Check sheet for the modelled part. Datum: model origin and axes. Units: mm. Round coordinates to 2 decimals unless told otherwise and drop trailing zeros. Order: outer loops, then holes, each group sorted by start corner. A loop starts at its lowest first (then second) coordinate and runs counter-clockwise, first axis right, second up.
(1) Sectioned sample at A-A, the plane y = 4. Enter the section's corners in (x, z).
(2) Depth check by flat-ended pin: pin 1 (8 mm diameter, centred on y = 4.5, z = 760.5, fed in from +X); pin 2 (8 mm diameter, centred on x = 18, z = 262.5, fed in from -Y); pin 3 (1 mm diameter, centred on x = 16, z = 714, fed in from +Y). Enter the tip coordinate at first touch or a pass-through.
(3) Thickness scan on probe 1 along Z at (x, y) = (38, 0.5); probe 2 along Z at (x, y) = (4, -6); probe 3 along Z at (x, y) = (30, -5.5). Record the ranges inside material, lowest first.
```python
from build123d import *

# Parameters (mm, degrees)
F0_W         = 20
F0_H         = 1249.13
F0_W_2       = 50
F0_H_2       = 16
F0_H_3       = 2
F1_DEPTH     = 10
F0_H_4       = 19
F2_DEPTH     = 11.5
F3_DEPTH     = 9.5
F4_DEPTH     = 8
F5_R         = 7.99999
F6_R         = 9.49999
F7_T1_DEPTH  = 107.4995000022
F7_T6_DEPTH  = 107.4995000022
F7_T12_DEPTH = 107.4995000022
F7_T18_DEPTH = 107.4995000022
F7_T25_DEPTH = 107.4995000022
F7_T31_DEPTH = 107.4995000022
F7_T37_DEPTH = 107.4995000022
F7_T43_DEPTH = 107.4995000022
F7_T49_DEPTH = 107.4995000022
F7_T56_DEPTH = 107.4995000022
F7_T62_DEPTH = 107.4995000022
F8_R         = 9.99999


# Not quite as in the source:
# - a fillet or chamfer that OpenCascade refuses, or shapes differently, is made with other operations: its cross-section is extruded or revolved along the edge and cut away or added
# - a fillet or chamfer is up to 0.001 mm smaller than in the source, because OpenCascade refuses the exact size


with BuildPart() as f1:
    # F0 (on Front) → F1 (new body, symmetric)
    with BuildSketch(Plane.XZ):
        with Locations((25, 647.565)):
            Rectangle(F0_W, F0_H)
        Polygon((0, 1272.13), (15, 1272.13), (35, 1272.13), (50, 1272.13), (50, 1274.13), (0, 1274.13), align=None)
        with Locations((25, 1282.13)):
            Rectangle(F0_W_2, F0_H_2)
        with Locations((25, 1291.13)):
            Rectangle(F0_W_2, F0_H_3)
    extrude(amount=F1_DEPTH, both=True)

    # F0 (on Front) → F2 (join, symmetric)
    with BuildSketch(Plane.XZ):
        Polygon((0, 23), (0, 21), (50, 21), (50, 23), (35, 23), (15, 23), align=None)
        with Locations((25, 11.5)):
            Rectangle(F0_W_2, F0_H_4)
        with Locations((25, 1)):
            Rectangle(F0_W_2, F0_H_3)
    extrude(amount=F2_DEPTH, both=True)

    # F0 (on Front) → F3 (cut, symmetric)
    with BuildSketch(Plane.XZ):
        with Locations((25, 11.5)):
            Rectangle(F0_W_2, F0_H_4)
    extrude(amount=F3_DEPTH, both=True, mode=Mode.SUBTRACT)

    # F0 (on Front) → F4 (cut, symmetric)
    with BuildSketch(Plane.XZ):
        with Locations((25, 1282.13)):
            Rectangle(F0_W_2, F0_H_2)
    extrude(amount=F4_DEPTH, both=True, mode=Mode.SUBTRACT)

    # F5 (radius 8 in the source; OpenCascade refuses exactly that, so slightly less here)
    f5_edges = [f1.edges().sort_by_distance(p)[0] for p in [
        (25, -8, 1290.13),
        (25, -8, 1274.13),
        (25, 8, 1274.13),
        (25, 8, 1290.13),
    ]]
    fillet(f5_edges, radius=F5_R)

    # F6 (radius 9.5 in the source; OpenCascade refuses exactly that, so slightly less here)
    f6_edges = [f1.edges().sort_by_distance(p)[0] for p in [
        (25, 9.5, 2),
        (25, -9.5, 2),
        (25, -9.5, 21),
        (25, 9.5, 21),
    ]]
    fillet(f6_edges, radius=F6_R)

    # F7: fillet of radius 11.5 on 4 edges, made by hand

    # F7_s2 → F7_t1 (cut)
    with BuildSketch(Plane.YZ.offset(-28.7497500011)):
        with BuildLine():
            ThreePointArc((-0.0001, -0.0001), (-8.1318279836, 3.3681720164), (-11.5001, 11.4999))
            Line((-11.5001, 11.4999), (-11.7301, 11.4999))
            ThreePointArc((-11.7301, 11.4999), (-11.73, 5.74995), (-11.73, 0))
            Line((-11.73, 0), (-11.5, -0.23))
            ThreePointArc((-11.5, -0.23), (-5.75005, -0.23), (-0.0001, -0.2301))
            Line((-0.0001, -0.2301), (-0.0001, -0.0001))
        make_face()
        with BuildLine():
            ThreePointArc((0.0001, -0.0001), (8.1318279836, 3.3681720164), (11.5001, 11.4999))
            Line((11.5001, 11.4999), (11.7301, 11.4999))
            ThreePointArc((11.7301, 11.4999), (11.73, 5.74995), (11.73, 0))
            Line((11.73, 0), (11.5, -0.23))
            ThreePointArc((11.5, -0.23), (5.75005, -0.23), (0.0001, -0.2301))
            Line((0.0001, -0.2301), (0.0001, -0.0001))
        make_face()
    extrude(amount=F7_T1_DEPTH, mode=Mode.SUBTRACT)


with BuildPart() as f7_tool4:
    # F7_s5 → F7_t6 (new body)
    with BuildSketch(Plane.YZ.offset(78.7497500011)):
        with BuildLine():
            ThreePointArc((-11.5001, 11.5001), (-8.1318279836, 19.6318279836), (-0.0001, 23.0001))
            Line((-0.0001, 23.0001), (-0.0001, 23.2301))
            ThreePointArc((-0.0001, 23.2301), (-5.75005, 23.23), (-11.5, 23.23))
            Line((-11.5, 23.23), (-11.73, 23))
            ThreePointArc((-11.73, 23), (-11.73, 17.25005), (-11.7301, 11.5001))
            Line((-11.7301, 11.5001), (-11.5001, 11.5001))
        make_face()
    extrude(amount=-F7_T6_DEPTH)

    split(bisect_by=Plane.XZ.offset(10), keep=Keep.TOP)

    split(bisect_by=Plane.YZ.offset(35), keep=Keep.TOP)


with BuildPart() as f1_1:
    add(f1.part)

    # F7_t3: cut F7_tool4
    add(f7_tool4.part, mode=Mode.SUBTRACT)


with BuildPart() as f7_tool10:
    # F7_s11 → F7_t12 (new body)
    with BuildSketch(Plane.YZ.offset(78.7497500011)):
        with BuildLine():
            ThreePointArc((-11.5001, 11.5001), (-8.1318279836, 19.6318279836), (-0.0001, 23.0001))
            Line((-0.0001, 23.0001), (-0.0001, 23.2301))
            ThreePointArc((-0.0001, 23.2301), (-5.75005, 23.23), (-11.5, 23.23))
            Line((-11.5, 23.23), (-11.73, 23))
            ThreePointArc((-11.73, 23), (-11.73, 17.25005), (-11.7301, 11.5001))
            Line((-11.7301, 11.5001), (-11.5001, 11.5001))
        make_face()
    extrude(amount=-F7_T12_DEPTH)

    split(bisect_by=Plane.XZ.offset(10), keep=Keep.BOTTOM)

    split(bisect_by=Plane.YZ.offset(35), keep=Keep.TOP)


with BuildPart() as f1_2:
    add(f1_1.part)

    # F7_t9: cut F7_tool10
    add(f7_tool10.part, mode=Mode.SUBTRACT)


with BuildPart() as f7_tool16:
    # F7_s17 → F7_t18 (new body)
    with BuildSketch(Plane.YZ.offset(78.7497500011)):
        with BuildLine():
            ThreePointArc((-11.5001, 11.5001), (-8.1318279836, 19.6318279836), (-0.0001, 23.0001))
            Line((-0.0001, 23.0001), (-0.0001, 23.2301))
            ThreePointArc((-0.0001, 23.2301), (-5.75005, 23.23), (-11.5, 23.23))
            Line((-11.5, 23.23), (-11.73, 23))
            ThreePointArc((-11.73, 23), (-11.73, 17.25005), (-11.7301, 11.5001))
            Line((-11.7301, 11.5001), (-11.5001, 11.5001))
        make_face()
    extrude(amount=-F7_T18_DEPTH)

    split(bisect_by=Plane.YZ.offset(15), keep=Keep.TOP)

    split(bisect_by=Plane.XZ.offset(10), keep=Keep.TOP)

    split(bisect_by=Plane.YZ.offset(35), keep=Keep.BOTTOM)


with BuildPart() as f1_3:
    add(f1_2.part)

    # F7_t15: cut F7_tool16
    add(f7_tool16.part, mode=Mode.SUBTRACT)


with BuildPart() as f7_tool23:
    # F7_s24 → F7_t25 (new body)
    with BuildSketch(Plane.YZ.offset(78.7497500011)):
        with BuildLine():
            ThreePointArc((-11.5001, 11.5001), (-8.1318279836, 19.6318279836), (-0.0001, 23.0001))
            Line((-0.0001, 23.0001), (-0.0001, 23.2301))
            ThreePointArc((-0.0001, 23.2301), (-5.75005, 23.23), (-11.5, 23.23))
            Line((-11.5, 23.23), (-11.73, 23))
            ThreePointArc((-11.73, 23), (-11.73, 17.25005), (-11.7301, 11.5001))
            Line((-11.7301, 11.5001), (-11.5001, 11.5001))
        make_face()
    extrude(amount=-F7_T25_DEPTH)

    split(bisect_by=Plane.YZ.offset(15), keep=Keep.BOTTOM)

    split(bisect_by=Plane.XZ.offset(10), keep=Keep.TOP)


with BuildPart() as f1_4:
    add(f1_3.part)

    # F7_t22: cut F7_tool23
    add(f7_tool23.part, mode=Mode.SUBTRACT)


with BuildPart() as f7_tool29:
    # F7_s30 → F7_t31 (new body)
    with BuildSketch(Plane.YZ.offset(78.7497500011)):
        with BuildLine():
            ThreePointArc((-11.5001, 11.5001), (-8.1318279836, 19.6318279836), (-0.0001, 23.0001))
            Line((-0.0001, 23.0001), (-0.0001, 23.2301))
            ThreePointArc((-0.0001, 23.2301), (-5.75005, 23.23), (-11.5, 23.23))
            Line((-11.5, 23.23), (-11.73, 23))
            ThreePointArc((-11.73, 23), (-11.73, 17.25005), (-11.7301, 11.5001))
            Line((-11.7301, 11.5001), (-11.5001, 11.5001))
        make_face()
    extrude(amount=-F7_T31_DEPTH)

    split(bisect_by=Plane.YZ.offset(15), keep=Keep.BOTTOM)

    split(bisect_by=Plane.XZ.offset(10), keep=Keep.BOTTOM)


with BuildPart() as f1_5:
    add(f1_4.part)

    # F7_t28: cut F7_tool29
    add(f7_tool29.part, mode=Mode.SUBTRACT)


with BuildPart() as f7_tool35:
    # F7_s36 → F7_t37 (new body)
    with BuildSketch(Plane.YZ.offset(78.7497500011)):
        with BuildLine():
            ThreePointArc((11.5001, 11.5001), (8.1318279836, 19.6318279836), (0.0001, 23.0001))
            Line((0.0001, 23.0001), (0.0001, 23.2301))
            ThreePointArc((0.0001, 23.2301), (5.75005, 23.23), (11.5, 23.23))
            Line((11.5, 23.23), (11.73, 23))
            ThreePointArc((11.73, 23), (11.73, 17.25005), (11.7301, 11.5001))
            Line((11.7301, 11.5001), (11.5001, 11.5001))
        make_face()
    extrude(amount=-F7_T37_DEPTH)

    split(bisect_by=Plane.YZ.offset(35), keep=Keep.TOP)

    split(bisect_by=Plane.XZ.offset(-10), keep=Keep.BOTTOM)


with BuildPart() as f1_6:
    add(f1_5.part)

    # F7_t34: cut F7_tool35
    add(f7_tool35.part, mode=Mode.SUBTRACT)


with BuildPart() as f7_tool41:
    # F7_s42 → F7_t43 (new body)
    with BuildSketch(Plane.YZ.offset(78.7497500011)):
        with BuildLine():
            ThreePointArc((11.5001, 11.5001), (8.1318279836, 19.6318279836), (0.0001, 23.0001))
            Line((0.0001, 23.0001), (0.0001, 23.2301))
            ThreePointArc((0.0001, 23.2301), (5.75005, 23.23), (11.5, 23.23))
            Line((11.5, 23.23), (11.73, 23))
            ThreePointArc((11.73, 23), (11.73, 17.25005), (11.7301, 11.5001))
            Line((11.7301, 11.5001), (11.5001, 11.5001))
        make_face()
    extrude(amount=-F7_T43_DEPTH)

    split(bisect_by=Plane.YZ.offset(35), keep=Keep.TOP)

    split(bisect_by=Plane.XZ.offset(-10), keep=Keep.TOP)


with BuildPart() as f1_7:
    add(f1_6.part)

    # F7_t40: cut F7_tool41
    add(f7_tool41.part, mode=Mode.SUBTRACT)


with BuildPart() as f7_tool47:
    # F7_s48 → F7_t49 (new body)
    with BuildSketch(Plane.YZ.offset(78.7497500011)):
        with BuildLine():
            ThreePointArc((11.5001, 11.5001), (8.1318279836, 19.6318279836), (0.0001, 23.0001))
            Line((0.0001, 23.0001), (0.0001, 23.2301))
            ThreePointArc((0.0001, 23.2301), (5.75005, 23.23), (11.5, 23.23))
            Line((11.5, 23.23), (11.73, 23))
            ThreePointArc((11.73, 23), (11.73, 17.25005), (11.7301, 11.5001))
            Line((11.7301, 11.5001), (11.5001, 11.5001))
        make_face()
    extrude(amount=-F7_T49_DEPTH)

    split(bisect_by=Plane.YZ.offset(15), keep=Keep.TOP)

    split(bisect_by=Plane.YZ.offset(35), keep=Keep.BOTTOM)

    split(bisect_by=Plane.XZ.offset(-10), keep=Keep.BOTTOM)


with BuildPart() as f1_8:
    add(f1_7.part)

    # F7_t46: cut F7_tool47
    add(f7_tool47.part, mode=Mode.SUBTRACT)


with BuildPart() as f7_tool54:
    # F7_s55 → F7_t56 (new body)
    with BuildSketch(Plane.YZ.offset(78.7497500011)):
        with BuildLine():
            ThreePointArc((11.5001, 11.5001), (8.1318279836, 19.6318279836), (0.0001, 23.0001))
            Line((0.0001, 23.0001), (0.0001, 23.2301))
            ThreePointArc((0.0001, 23.2301), (5.75005, 23.23), (11.5, 23.23))
            Line((11.5, 23.23), (11.73, 23))
            ThreePointArc((11.73, 23), (11.73, 17.25005), (11.7301, 11.5001))
            Line((11.7301, 11.5001), (11.5001, 11.5001))
        make_face()
    extrude(amount=-F7_T56_DEPTH)

    split(bisect_by=Plane.YZ.offset(15), keep=Keep.BOTTOM)

    split(bisect_by=Plane.XZ.offset(-10), keep=Keep.BOTTOM)


with BuildPart() as f1_9:
    add(f1_8.part)

    # F7_t53: cut F7_tool54
    add(f7_tool54.part, mode=Mode.SUBTRACT)


with BuildPart() as f7_tool60:
    # F7_s61 → F7_t62 (new body)
    with BuildSketch(Plane.YZ.offset(78.7497500011)):
        with BuildLine():
            ThreePointArc((11.5001, 11.5001), (8.1318279836, 19.6318279836), (0.0001, 23.0001))
            Line((0.0001, 23.0001), (0.0001, 23.2301))
            ThreePointArc((0.0001, 23.2301), (5.75005, 23.23), (11.5, 23.23))
            Line((11.5, 23.23), (11.73, 23))
            ThreePointArc((11.73, 23), (11.73, 17.25005), (11.7301, 11.5001))
            Line((11.7301, 11.5001), (11.5001, 11.5001))
        make_face()
    extrude(amount=-F7_T62_DEPTH)

    split(bisect_by=Plane.YZ.offset(15), keep=Keep.BOTTOM)

    split(bisect_by=Plane.XZ.offset(-10), keep=Keep.TOP)


with BuildPart() as f1_10:
    add(f1_9.part)

    # F7_t59: cut F7_tool60
    add(f7_tool60.part, mode=Mode.SUBTRACT)

    # F8 (radius 10 in the source; OpenCascade refuses exactly that, so slightly less here)
    f8_edges = [f1_10.edges().sort_by_distance(p)[0] for p in [
        (7.5, -10, 1272.13),
        (25, -10, 1292.13),
        (42.5, -10, 1272.13),
        (35, -10, 644.654592),
        (15, -10, 644.654592),
        (35, 10, 644.654592),
        (42.5, 10, 1272.13),
        (25, 10, 1292.13),
        (15, 10, 644.654592),
        (7.5, 10, 1272.13),
    ]]
    fillet(f8_edges, radius=F8_R)


solid = f1_10.part
```
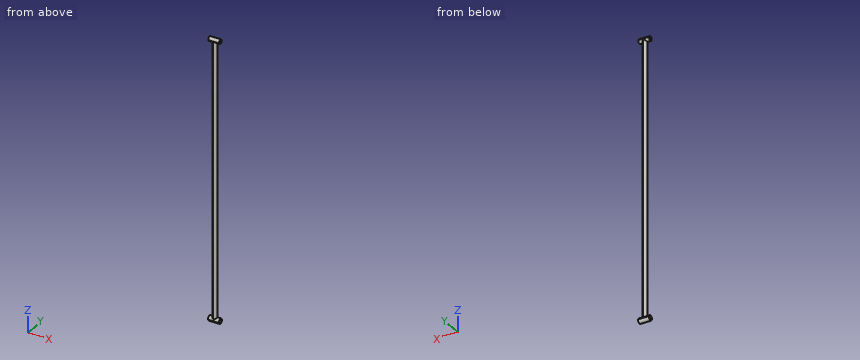
Derived:
1. outline: (0, 0.72) - (50, 0.72) - (50, 2.88) - (0, 2.88) - close; (0, 20.12) - (50, 20.12) - (50, 22.28) - (34.17, 22.28) - (34.17, 1272.96) - (50, 1272.96) - (50, 1275.2) - (0, 1275.2) - (0, 1272.96) - (15.83, 1272.96) - (15.83, 22.28) - (0, 22.28) - close; (0, 1289.06) - (50, 1289.06) - (50, 1291.3) - (0, 1291.3) - close
2. pin 1: stops at x = 34.99
2. pin 2: stops at y = -9.54
2. pin 3: stops at y = 5.27
3. probe 1: z = 0.01 to 2.01, 20.99 to 22.99, 1272.14 to 1274.15, 1290.11 to 1292.12
3. probe 2: z = 1.69 to 4.13, 18.87 to 21.31, 1274.13 to 1276.84, 1287.42 to 1290.13
3. probe 3: z = 1.4 to 3.75, 19.25 to 1276.32, 1287.94 to 1290.48
